```python
from build123d import *

# Parameters (mm, degrees)
F0_W     = 60.8845241368
F0_H     = 36.5624986589
F1_DEPTH = 25
F2_T     = -1
F3_R     = 5.8019318328
F3_R_2   = 5.7407936272
F4_DEPTH = 5.9
F5_DEPTH = 11.4
F6_T     = -2.5
F9_D     = 2
F10_R    = 2
F11_R    = 0.0241421356
F12_R    = 0.0241421356


# Not quite as in the source:
# - a feature of the source that left no trace in its solid (it failed there, or was rolled back) is left out


with BuildPart() as f1:
    # F0 (on Front) → F1 (new body)
    with BuildSketch(Plane.XZ):
        with Locations((-30.4422620684, -18.2812493294)):
            Rectangle(F0_W, F0_H)
    extrude(amount=F1_DEPTH)

    # F2
    f2_openings = [f1.faces().sort_by_distance(p)[0] for p in [
        (0, -12.5, -18.281249),
    ]]
    offset(amount=F2_T, openings=f2_openings)

    # F3 (on face) → F4 (join)
    with BuildSketch(Plane(origin=(-60.8845241368, 0, 0), x_dir=(0, -1, 0), z_dir=(-1, 0, 0))):
        with Locations((12.2040687129, -16.6244860739)):
            Circle(F3_R)
        with Locations((12.2040687129, -16.6244860739)):
            Circle(F3_R_2, mode=Mode.SUBTRACT)
    extrude(amount=F4_DEPTH)

    # F5 (add): a face of the model
    f5_faces = [f1.faces().sort_by_distance(p)[0] for p in [
        (-60.8845241368, -12.2040687129, -16.6244860739),
    ]]
    extrude(f5_faces, amount=-F5_DEPTH)

    # F6
    f6_openings = [f1.faces().sort_by_distance(p)[0] for p in [
        (-49.484524, -12.204069, -16.624486),
    ]]
    offset(amount=F6_T, openings=f6_openings)

    # F9 (through all)
    with Locations(Plane(origin=(-60.8845241368, 0, 0), x_dir=(0, -1, 0), z_dir=(-1, 0, 0))):
        with Locations((12.2040687129, -16.6244860739)):
            Hole(F9_D / 2)

    # F10
    f10_edges = [f1.edges().sort_by_distance(p)[0] for p in [
        (-30.442262, -25, -36.562499),
        (-30.442262, -25, 0),
    ]]
    fillet(f10_edges, radius=F10_R)

    # F11
    f11_edges = [f1.edges().sort_by_distance(p)[0] for p in [
        (-30.442262, 0, -36.562499),
        (-30.442262, 0, 0),
    ]]
    fillet(f11_edges, radius=F11_R)

    # F12
    f12_edges = [f1.edges().sort_by_distance(p)[0] for p in [
        (-30.442262, -0.024142, -36.562499),
        (-30.442262, 0, -0.024142),
        (0, 0, -18.281249),
        (-60.884524, 0, -18.281249),
        (0, -11.512071, 0),
        (-60.884524, -11.512071, 0),
        (0, -11.512071, -36.562499),
        (0, -0.007071, -36.555428),
        (0, -24.414214, -35.976712),
        (0, -25, -18.281249),
        (0, -0.007071, -0.007071),
        (0, -24.414214, -0.585786),
        (-60.884524, -0.007071, -0.007071),
        (-60.884524, -24.414214, -0.585786),
        (-60.884524, -25, -18.281249),
        (-60.884524, -0.007071, -36.555428),
        (-60.884524, -24.414214, -35.976712),
        (-60.884524, -11.512071, -36.562499),
    ]]
    fillet(f12_edges, radius=F12_R)


solid = f1.part
```
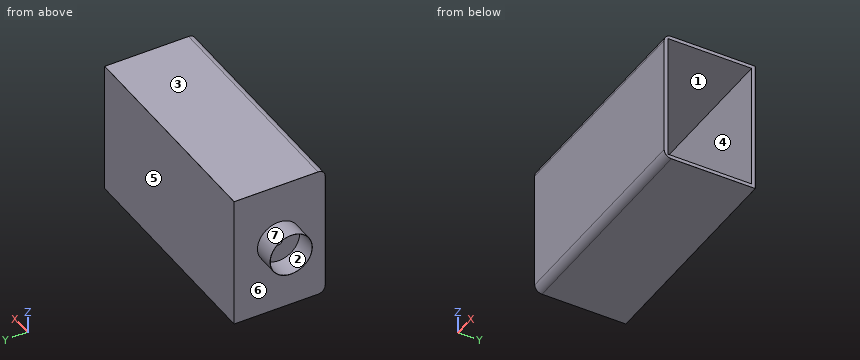
Input: part model. Units: mm. Frame: model coordinates. Face numbers are marked on the shaded views. A direction names the side the tool comes from. Coordinates: 2 decimals unless noted, no trailing zeros.
1) Set-up query: the marked faces 1, 2 and 3. Return all of +Z, -Z, +X, -X, +Y, -Y with unobstructed straight access to the full face (end or side cutting, diameter ignored); none if empty.
2) Mould query, pull axis Y, two halves, no side actions, for the marked faces 4, 5, 6 and 7. Classes: pulls with the +Y half, pulls with the -Y half, needs draft (parallel to the pull), parting line crosses it, or undercut.
3) Section A-A on x = -56.5. State how many separate pieces and enclosed holes the cut face has, and give its area (3 significant figures).
4) Material intervals for line 1 along Z through (x, y) = (-3.5, -19.5); line 2 along Y through (x, z) = (-36.5, -23); line 3 along Y through (x, z) = (-55.5, -21), sorted ascending.
5) Pin query (flat end, axial travel): pin 1 Ø7 at (y, z) = (-17, -16) entering from +X; pin 2 Ø2.5 at (y, z) = (-12.2, -16.62) entering from -X; pin 3 Ø4 at (y, z) = (-15, -30.5) entering from +X. Return the tip coordinate at first contact, or that it passes through.
Check result:
1. face 1: +X
1. face 2: -X
1. face 3: +Z, +X, -X, +Y, -Y
2. face 4: undercut
2. face 5: pulls with the +Y half
2. face 6: needs draft
2. face 7: parting line crosses it
3. separate pieces: 2
3. enclosed holes: 2
3. area: 188 mm2
4. line 1: z = -36.56 to -35.56, -1 to 0
4. line 2: y = -25 to -24, -1 to 0
4. line 3: y = -25 to -24, -15.92 to -8.49, -1 to 0
5. pin 1: stops at x = -49.48
5. pin 2: stops at x = -60.88
5. pin 3: stops at x = -59.88
